from build123d import *

# Parameters (mm, degrees)
SKETCH1_W                     = 127
SKETCH1_H                     = 82.55
PLATE_DEPTH                   = 6.35
BEARING_NUT_HELICOIL_HOLES_D  = 5.1054
ROUTER_MOUNT_HELICOIL_HOLES_D = 5.1054


with BuildPart() as part:
    # Sketch1 → Plate (new body)
    with BuildSketch(Plane.XY):
        Rectangle(SKETCH1_W, SKETCH1_H)
    extrude(amount=PLATE_DEPTH)

    # Bearing/Nut Helicoil Holes (through all)
    with Locations(Plane(origin=(0, 0, 0), x_dir=(-1, 0, 0), z_dir=(0, 0, -1))):
        with Locations((-56.3565, 7.9375), (-19.844, -14.2875), (-56.3565, -14.2875), (-19.844, 7.9375), (19.844, 7.9375), (56.3565, -14.2875), (19.844, -14.2875), (56.3565, 7.9375), (-19.05, 28.575), (19.05, 28.575)):
            Hole(BEARING_NUT_HELICOIL_HOLES_D / 2)

    # Router Mount Helicoil Holes (through all)
    with Locations(Plane(origin=(0, 0, 0), x_dir=(-1, 0, 0), z_dir=(0, 0, -1))):
        with Locations((-47.625, 25.4), (47.625, -25.4), (-47.625, -25.4), (47.625, 25.4)):
            Hole(ROUTER_MOUNT_HELICOIL_HOLES_D / 2)


solid = part.part
Could you check a few things on this model? Use its own coordinates, in mm. Coordinates: 2 decimals unless noted, no trailing zeros. Order: outer loops, then holes, each group sorted by start corner. A loop starts at its lowest first (then second) coordinate and runs counter-clockwise, first axis right, second up. Notation, with made-up numbers: (86.25, 53) -> (95.25, 53) arc R34 ccw to (95.25, 84) -> close; hole circle Ø4 at (-26, 70.25). An arc over 180 degrees is marked (long way). One line per question, with ' | ' between items.
Q1. Imagine slicing it at D-D on x = 20. Please give me the cut outline in (y, z) (3 decimals).
Return value:
outline: (-41.275, 0) -> (-16.835, 0) -> (-16.835, 6.35) -> (-41.275, 6.35) -> close; (-11.74, 0) -> (5.39, 0) -> (5.39, 6.35) -> (-11.74, 6.35) -> close; (10.485, 0) -> (26.206, 0) -> (26.206, 6.35) -> (10.485, 6.35) -> close; (30.944, 0) -> (41.275, 0) -> (41.275, 6.35) -> (30.944, 6.35) -> close
Q2. Imagine slicing it at C-C on z = 1.5. State how many separate pieces and enclosed holes the cut face has, and give its area (3 significant figures).
Return value:
separate pieces: 1 | enclosed holes: 14 | area: 10,200 mm²
Q3. If I drill on L1, parallel to X at y = -14, z = 3.25; L2, parallel to Y at x = 57, z = 2.5 (3 decimals); L3, parallel to X at y = 27, z = 1.5, over which ranges is the centre line in solid material (lowest first)?
Return value:
L1: -63.5 to -58.89, -53.82 to -22.38, -17.31 to 17.31, 22.38 to 53.82, 58.89 to 63.5 | L2: -41.275 to -16.758, -11.817 to 5.467, 10.408 to 41.275 | L3: -63.5 to -49.61, -45.64 to -21.06, -17.04 to 17.04, 21.06 to 45.64, 49.61 to 63.5
Q4. Thinking about a two-plate mould opening in Y: for faces 1 (the face through (-53.92, 8.7, 3.22)), 2 (the face through (-1, -41.275, 3)), 3 (the face through (-1, 1, 0)), which applies, pulls with the +Y half, pulls with the -Y half, needs draft (parallel to the pull), parting line crosses it, or undercut?
Return value:
face 1: undercut | face 2: pulls with the -Y half | face 3: needs draft
Q5. Imagine slicing it at B-B on x = -19.05. Please give me the cut outline in (y, z) (3 decimals), and give its area (3 significant figures).
Return value:
outline: (-41.275, 0) -> (-16.714, 0) -> (-16.714, 6.35) -> (-41.275, 6.35) -> close; (-11.861, 0) -> (5.511, 0) -> (5.511, 6.35) -> (-11.861, 6.35) -> close; (10.364, 0) -> (26.022, 0) -> (26.022, 6.35) -> (10.364, 6.35) -> close; (31.128, 0) -> (41.275, 0) -> (41.275, 6.35) -> (31.128, 6.35) -> close | area: 430 mm²
Q6. Imagine slicing it at A-A on y = -25.4. Please give me the cut outline in (x, z).
Return value:
outline: (-63.5, 0) -> (-50.18, 0) -> (-50.18, 6.35) -> (-63.5, 6.35) -> close; (-45.07, 0) -> (45.07, 0) -> (45.07, 6.35) -> (-45.07, 6.35) -> close; (50.18, 0) -> (63.5, 0) -> (63.5, 6.35) -> (50.18, 6.35) -> close
